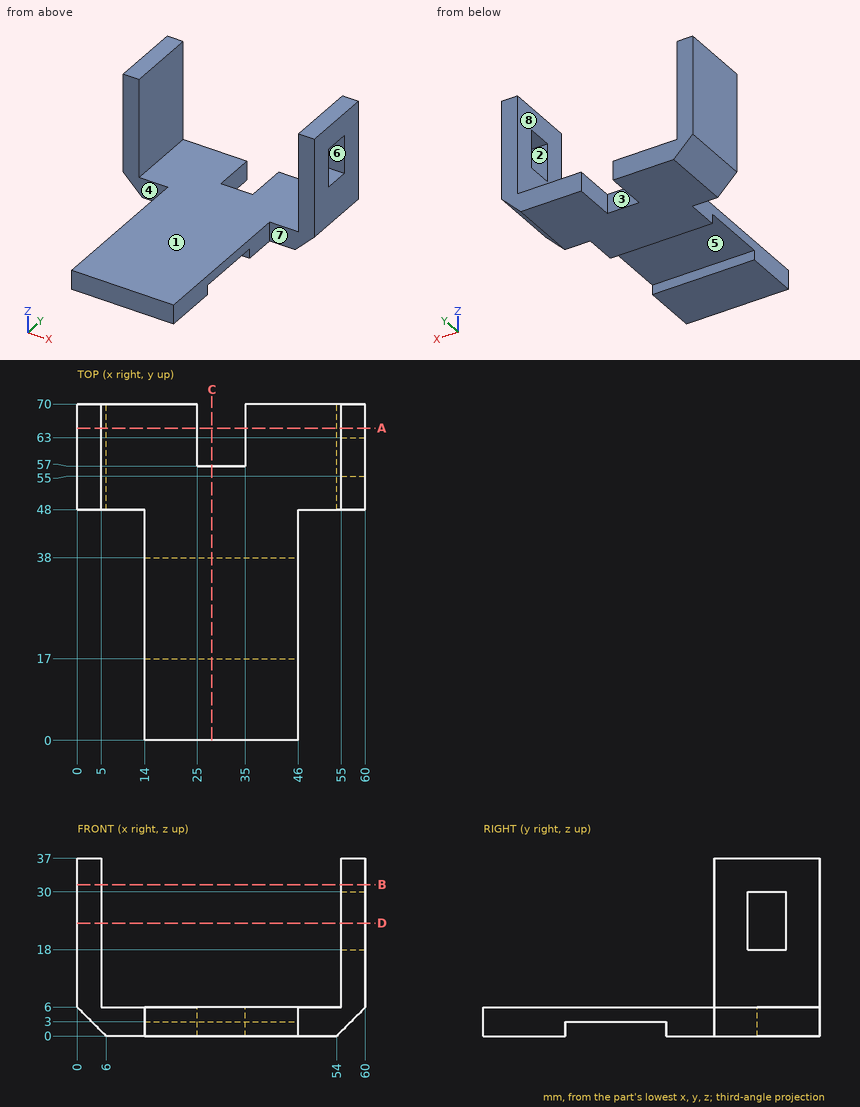
Design review of the part shown in the three views and the two pictorial views. Dimensions are in mm from the part's minimum x, y and z. A direction names the side the tool comes from. Coordinates: 2 decimals unless noted, no trailing zeros. Loops run counter-clockwise (first coordinate to the right, second up) from the corner with the lowest first, then second, coordinate; pieces in that order, holes last. Notation, with made-up numbers: M 77,60.25 L 94,60.25 A16 ccw 94,72.25 Z; hole C 8.5,53.5 d7. An arc over 180 degrees is marked long. One line per question, with ' | ' between items.
(1) For pin 1 Ø6 at (y, z) = (47.5, 32) entering from -X; pin 2 Ø12 at (x, y) = (37.5, 27.5) entering from +Z; pin 3 Ø1.8 at (x, z) = (32, 3) entering from +Y; pin 4 Ø5 at (y, z) = (12, 2) entering from +X, all flat-tipped, find the tip position at first contact; note any pin that passes through.
Filled in:
pin 1: stops at x = 0 | pin 2: stops at z = 6 | pin 3: stops at y = 57 | pin 4: stops at x = 46
(2) We need section A-A (y = 65). Give the boundary of the cut face in (x, z).
Filled in:
outline: M 0,6 L 6,0 L 25,0 L 25,6 L 5,6 L 5,37 L 0,37 Z; M 35,0 L 54,0 L 60,6 L 60,37 L 55,37 L 55,6 L 35,6 Z
(3) Wall thickness on probe 1 along X at (y, z) = (57, 33.5); probe 2 along Z at (x, y) = (35.5, 39); probe 3 along Y at (x, z) = (55.5, 32): over which ranges is each line inside the solid? List them lowest first.
Filled in:
probe 1: x = 0 to 5, 55 to 60 | probe 2: z = 0 to 6 | probe 3: y = 48 to 70
(4) Draft analysis for pull direction Y (two halves, no side actions). For the marked faces 6, 7 and 8, state which applies: released by +Y, released by -Y, zero draft, split by the parting line, or undercut.
Filled in:
face 6: undercut | face 7: released by -Y | face 8: zero draft
(5) Machinability: for the marked faces 1, 2, 3, 4 and 5, which of the approach directions +Z, -Z, +X, -X, +Y, -Y give a long, thin tool a straight path to every point of the face, cutting with its end or side? Answer none if there is none.
Filled in:
face 1: +Z, +Y, -Y | face 2: +X | face 3: +Z, -Z, +Y | face 4: +Z, -Z, -X, -Y | face 5: -Z, +X, -X
(6) We need section C-C (x = 28). Give the boundary of the cut face in (y, z), and give its area (3 significant figures).
Filled in:
outline: M 0,0 L 17,0 L 17,3 L 38,3 L 38,0 L 57,0 L 57,6 L 0,6 Z | area: 279 mm^2
(7) We need section D-D (z = 23.5). Give the boundary of the cut face in (x, y).
Filled in:
outline: M 0,48 L 5,48 L 5,70 L 0,70 Z; M 55,48 L 60,48 L 60,55 L 55,55 Z; M 55,63 L 60,63 L 60,70 L 55,70 Z
(8) We need section B-B (z = 31.5). Give the boundary of the cut face in (x, y), and give its area (3 significant figures).
Filled in:
outline: M 0,48 L 5,48 L 5,70 L 0,70 Z; M 55,48 L 60,48 L 60,70 L 55,70 Z | area: 220 mm^2
